```python
from build123d import *

# Parameters (mm, degrees)
BOSS_EXTRUDE1_DEPTH = 125


with BuildPart() as part:
    # Sketch1 → Boss-Extrude1 (new, symmetric)
    with BuildSketch(Plane.XY):
        with BuildLine():
            Line((0, 4.1), (3.251471863, 4.1))
            Line((3.251471863, 4.1), (5.5, 6.348528137))
            Line((5.5, 6.348528137), (5.5, 8.4))
            Line((5.5, 8.4), (3.1, 8.4))
            Line((3.1, 8.4), (3.1, 9.5))
            Line((3.1, 9.5), (3.6, 10))
            Line((3.6, 10), (8.209994734, 10))
            ThreePointArc((8.209994734, 10), (8.895000093, 9.863743962), (9.475719596, 9.475719596))
            Line((9.475719596, 9.475719596), (1.767766953, 1.767766953))
            ThreePointArc((1.767766953, 1.767766953), (0.956708581, 2.309698831), (0, 2.5))
            Line((0, 2.5), (0, 4.1))
        make_face()
    extrude(amount=BOSS_EXTRUDE1_DEPTH, both=True)

    # Mirror1: part across plane


with BuildPart() as part_1:
    add(part.part)
    add(part.part.mirror(Plane(origin=(1.767766953, 1.767766953, 125), x_dir=(0, 0, 1), z_dir=(-0.7071067811865499, 0.7071067811865451, 0))))

    # Mirror2: part across plane


with BuildPart() as part_2:
    add(part_1.part)
    add(part_1.part.mirror(Plane(origin=(0, 4.1, 125), x_dir=(0, 0, 1), z_dir=(1, 0, 0))))

    # Mirror3: part across plane


with BuildPart() as part_3:
    add(part_2.part)
    add(part_2.part.mirror(Plane(origin=(-4.1, 0, 125), x_dir=(0, 0, 1), z_dir=(0, 1, 0))))


solid = part_3.part
```
Source: CAD feature listing. Evaluate the final solid. Frame: model axes, mm. Round coordinates to 2 decimals unless told otherwise and drop trailing zeros. Put each result on its own line as item: value.
(1) Ray query, line 1 (Y direction, x = 7.75, z = 99); line 2 (X direction, y = 4.25, z = 109.5); line 3 (X direction, y = -4.5, z = 49). Return the intervals inside material, ascending. Write a range as [from, to].
Solutions:
line 1: [-10, -5.5], [5.5, 10]
line 2: [-10, -8.4], [-5.1, -3.4], [3.4, 5.1], [8.4, 10]
line 3: [-10, -8.4], [-5.35, -3.65], [3.65, 5.35], [8.4, 10]
(2) First-contact query: pin 1 (1 mm diameter, centred on y = -0.5, z = -72, fed in from +X); pin 2 (0.9 mm diameter, centred on y = 9, z = 60.5, fed in from -X); pin 3 (1.5 mm diameter, centred on y = -2.5, z = -86.5, fed in from -X); pin 4 (7 mm diameter, centred on x = -0.5, z = -33, fed in from +Y). Flat tips, straight axial feed; report the tip coordinate or a pass-through.
Solutions:
pin 1: x = 4.1
pin 2: x = -9.97
pin 3: x = -9.65
pin 4: y = 10
(3) Pull-direction query (Y, two-part tool) for faces 1 (the face through (6, 10, 2)), 2 (the face through (10, 6, 2)), 3 (the face through (4.1, 0, 2)); classes: released by +Y, released by -Y, zero draft, split by the parting line, or undercut.
Solutions:
face 1: released by +Y
face 2: zero draft
face 3: undercut
